The drawing under review shows one solid part. Ordinate dimensions are in mm from its lowest x, y, z. Coordinates: 2 decimals unless noted, no trailing zeros. Loops run counter-clockwise (first coordinate to the right, second up) from the corner with the lowest first, then second, coordinate; pieces in that order, holes last.
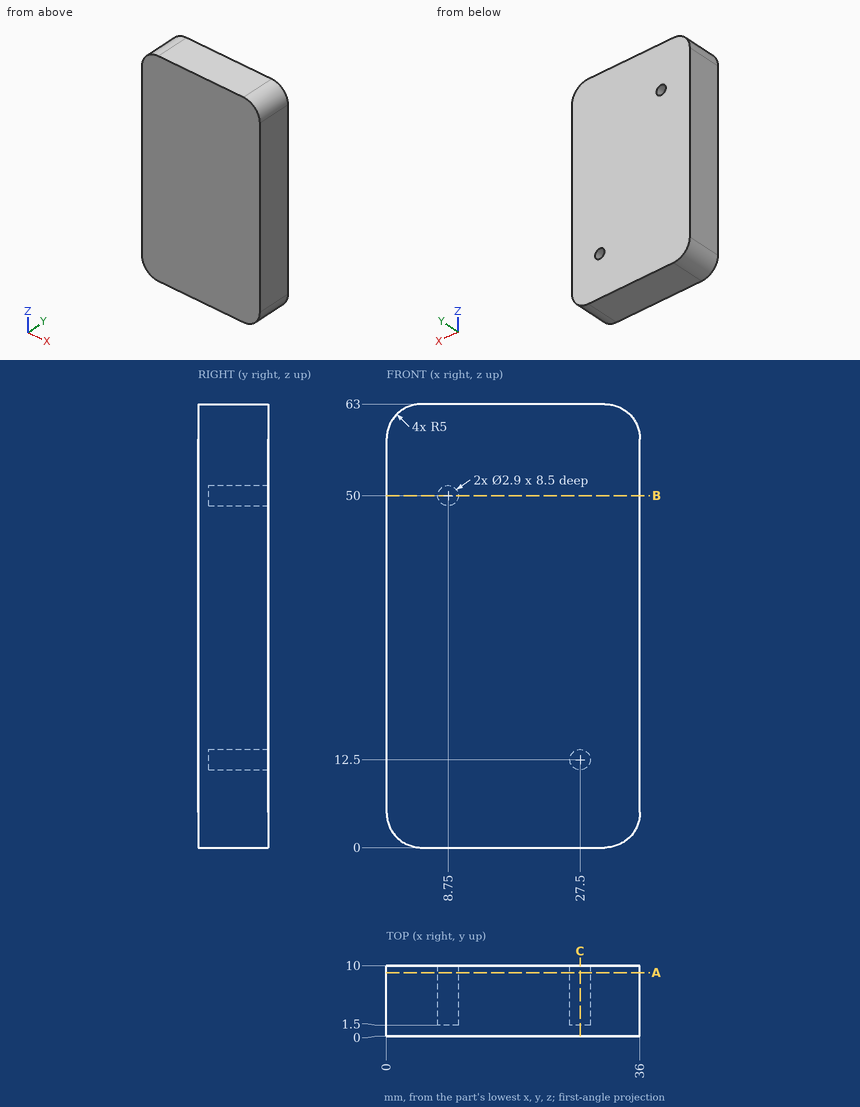
Q1. Take a section at C-C, the plane x = 27.5. Write out the cut boundary in (y, z), then the cut area to 3 significant figures.
Q2. Take a section at B-B, the plane z = 50. Write out the cut boundary in (x, y).
Q3. For line 1 (Z direction, x = 8.75, y = 4.5); line 2 (X direction, y = 4, z = 50); line 3 (Z direction, x = 27.5, y = 8.5), list the stretches that pass through material, from the lowest coordinate up.
Q4. Take a section at A-A, the plane y = 9. Write out the cut boundary in (x, z), then the cut area to 3 significant figures.
Q5. Clearance check with flat-ended pins moving along their axes: pin 1 Ø8 at (x, z) = (15.5, 23.5) entering from -Y; pin 2 Ø0.9 at (x, z) = (28, 12.5) entering from +Y. State where each tip first meets the part, or that it passes through.
Entries:
1. outline: (0, 0) - (10, 0) - (10, 11.05) - (1.5, 11.05) - (1.5, 13.95) - (10, 13.95) - (10, 63) - (0, 63) - close
1. area: 605 mm2
2. outline: (0, 0) - (36, 0) - (36, 10) - (10.2, 10) - (10.2, 1.5) - (7.3, 1.5) - (7.3, 10) - (0, 10) - close
3. line 1: z = 0 to 48.55, 51.45 to 63
3. line 2: x = 0 to 7.3, 10.2 to 36
3. line 3: z = 0 to 11.05, 13.95 to 63
4. outline: (0, 5) arc R5 ccw to (5, 0) - (31, 0) arc R5 ccw to (36, 5) - (36, 58) arc R5 ccw to (31, 63) - (5, 63) arc R5 ccw to (0, 58) - close; hole circle Ø2.9 at (8.75, 50); hole circle Ø2.9 at (27.5, 12.5)
4. area: 2,230 mm2
5. pin 1: stops at y = 0
5. pin 2: stops at y = 1.5
